Can you work these out from the model? Positions are in its coordinate system, mm. Face numbers are marked on the shaded views. A direction names the side the tool comes from. Coordinates: 2 decimals unless noted, no trailing zeros. Write each loop counter-clockwise with the first axis right and the second up, starting at its lowest first coordinate (ties: lowest second). Pieces come first, ordered by that corner, then holes. Notation, with made-up numbers: (-22.75, 35.25) -> (27.25, 35.25) arc R13 ccw to (27.25, 51.25) -> close; hole circle Ø8 at (10, 75.5). An arc over 180 degrees is marked (long way). Use one line per item in the form item = value.
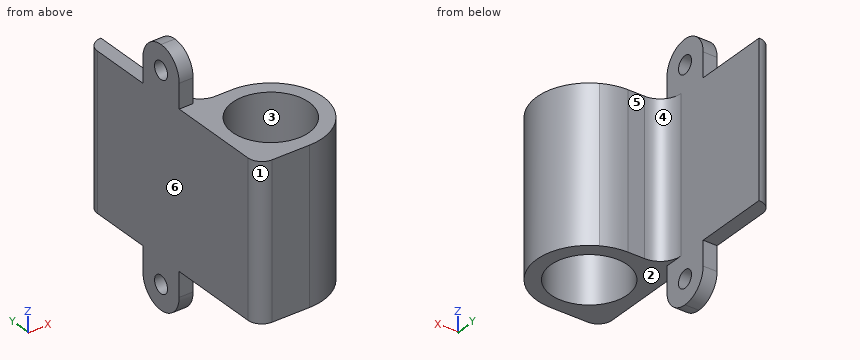
```python
from build123d import *

# Parameters (mm, degrees)
SKETCH2_R            = 11
BOSS_EXTRUDE1_DEPTH  = 44
SKETCH5_W            = 4
SKETCH5_H            = 14
BOSS_EXTRUDE3_DEPTH  = 14
FILLET3_R            = 7
SKETCH6_R            = 2.5
CUT_EXTRUDE2_DEPTH   = 14
FILLET3_OF_MIRROR2_R = 7


with BuildPart() as part:
    # Sketch2 → Boss-Extrude1 (new body)
    with BuildSketch(Plane.XY):
        with BuildLine():
            Line((0, 4), (0, 62))
            ThreePointArc((0, 62), (1.171572875, 64.828427125), (4, 66))
            Line((4, 66), (4, 36))
            ThreePointArc((4, 36), (5.757359313, 31.757359313), (10, 30))
            Line((10, 30), (14.75, 30))
            ThreePointArc((14.75, 30), (18.324268314, 29.567930739), (21.692625765, 28.296614136))
            ThreePointArc((21.692625765, 28.296614136), (29.317930739, 11.425731686), (14.75, 0))
            Line((14.75, 0), (4, 0))
            ThreePointArc((4, 0), (1.171572875, 1.171572875), (0, 4))
        make_face()
        with Locations((14.75, 15)):
            Circle(SKETCH2_R, mode=Mode.SUBTRACT)
    extrude(amount=BOSS_EXTRUDE1_DEPTH)

    # Sketch5 → Boss-Extrude3 (add)
    with BuildSketch(Plane.XY.offset(44)):
        with Locations((2, 37.473717009)):
            Rectangle(SKETCH5_W, SKETCH5_H)
    boss_extrude3 = extrude(amount=BOSS_EXTRUDE3_DEPTH)

    # Fillet3
    fillet3_edges = [part.edges().sort_by_distance(p)[0] for p in [
        (2, 30.473717009, 58),
        (2, 44.473717009, 58),
    ]]
    fillet(fillet3_edges, radius=FILLET3_R - 0.0001)  # a hair under: the kernel refuses the full size

    # Sketch6 → Cut-Extrude2 (cut)
    with BuildSketch(Plane(origin=(4, 0, 0), x_dir=(0, 0, -1), z_dir=(1, 0, 0))):
        with Locations(Location((-51, 37.473717009, 0), (0, 0, 90))):
            Circle(SKETCH6_R)
    cut_extrude2 = extrude(amount=-CUT_EXTRUDE2_DEPTH, mode=Mode.SUBTRACT)

    # Mirror2: Boss-Extrude3, Cut-Extrude2 across plane
    add(boss_extrude3.mirror(Plane(origin=(0, 0, 22), x_dir=(1, 0, 0), z_dir=(0, 0, -1))))
    add(cut_extrude2.mirror(Plane(origin=(0, 0, 22), x_dir=(1, 0, 0), z_dir=(0, 0, -1))), mode=Mode.SUBTRACT)

    # Fillet3 of Mirror2
    fillet3_of_mirror2_edges = [part.edges().sort_by_distance(p)[0] for p in [
        (2, 30.473717009, -14),
        (2, 44.473717009, -14),
    ]]
    fillet(fillet3_of_mirror2_edges, radius=FILLET3_OF_MIRROR2_R - 0.0001)  # a hair under: the kernel refuses the full size


solid = part.part
```
Q1. For the marked faces 5 and 6, which set-ups out of +Z, -Z, +X, -X, +Y, -Y let a thin tool reach every point of the face, with its end or its side?
Return value:
face_5 = +Z, -Z, +X, +Y
face_6 = +Z, -Z, -X, +Y, -Y
Q2. Suppose I cut it at B-B (z = 18). Write out the boundary of the cut face in (x, y), then the cut area to 3 significant figures.
Return value:
outline = (0, 4) arc R4 ccw to (4, 0) -> (14.75, 0) arc R15 ccw to (14.75, 30) -> (10, 30) arc R6 cw to (4, 36) -> (4, 66) arc R4 ccw to (0, 62) -> close; hole circle Ø22 at (14.75, 15)
area = 561 mm2
Q3. Thinking about a two-plate mould opening in Y: for the marked faces 1, 2, 3 and 4, which applies, released by +Y, released by -Y, zero draft, split by the parting line, or undercut?
Return value:
face_1 = released by -Y
face_2 = zero draft
face_3 = undercut
face_4 = released by +Y
Q4. Suppose I cut it at D-D (z = -1.5). Write out the boundary of the cut face in (x, y).
Return value:
outline = (0, 30.47) -> (4, 30.47) -> (4, 44.47) -> (0, 44.47) -> close
Q5. Will these pins go through, and if not, where does the flat tip stop? pin 1 (1.2 mm diameter, centred on x = 1.5, z = -3.5, fed in from +Y); pin 2 (8 mm diameter, centred on y = 40.5, z = 36, fed in from +X); pin 3 (8 mm diameter, centred on y = 37.47, z = 51, fed in from -X); pin 4 (3 mm diameter, centred on y = 37.47, z = -7, fed in from -X).
Return value:
pin_1 = 44.47
pin_2 = 4
pin_3 = 0
pin_4 = through
Q6. If I drill on line 1 (Y direction, x = 2.85, z = -7); line 2 (X direction, y = 61.5, z = 0.5); line 3 (Z direction, x = 23.5, y = 3.5), over which ranges is the centre line in solid material (lowest first)? Write a range as from..to.
Return value:
line_1 = 30.47..34.97, 39.97..44.47
line_2 = 0..4
line_3 = 0..44
Q7. Suppose I cut it at C-C (z = 52.5). Write out the boundary of the cut face in (x, y), then the cut area to 3 significant figures.
Return value:
outline = (0, 30.64) -> (4, 30.64) -> (4, 35.47) -> (0, 35.47) -> close; (0, 39.47) -> (4, 39.47) -> (4, 44.31) -> (0, 44.31) -> close
area = 38.7 mm2
Q8. Suppose I cut it at A-A (y = 15). Write out the boundary of the cut face in (x, z).
Return value:
outline = (0, 0) -> (3.75, 0) -> (3.75, 44) -> (0, 44) -> close; (25.75, 0) -> (29.75, 0) -> (29.75, 44) -> (25.75, 44) -> close
